Verification items for the finished model (mm, model axes). A direction names the side the tool comes from. Round coordinates to 2 decimals unless told otherwise and drop trailing zeros. Loops run counter-clockwise (first coordinate to the right, second up) from the corner with the lowest first, then second, coordinate; pieces in that order, holes last. Notation, with made-up numbers: (3.5, 25.25) -> (47.5, 25.25) arc R27 cw to (47.5, 57.25) -> close; hole circle Ø10 at (70.5, -29). An arc over 180 degrees is marked (long way). Write item = value, one per line.
```python
from build123d import *

# Parameters (mm, degrees)
BOSS_EXTRUDE1_DEPTH             = 20
SKETCH6_W                       = 25
SKETCH6_H                       = 20
BOSS_EXTRUDE5_DEPTH             = 5.5
BOSS_EXTRUDE11_START            = -20
BOSS_EXTRUDE11_DEPTH            = 34
SKETCH4_R                       = 2
CUT_EXTRUDE1_DEPTH              = 10
BOSS_EXTRUDE13_DEPTH            = 12
FILLET11_START                  = 14.0499999
FILLET11_DEPTH                  = 7.9500001
FILLET11_START_2                = -14.996842371
FILLET11_2_DEPTH                = 30.996842371
SKETCH22_R                      = 2
CUT_EXTRUDE6_DEPTH              = 10
CHAMFER1_SIZE                   = 14
SKETCH26_W                      = 22
SKETCH26_H                      = 20
BOSS_EXTRUDE14_DEPTH            = 11
CUT_EXTRUDE7_DEPTH              = 2.5
CUT_EXTRUDE8_REACH              = 65.92
SKETCH27_R                      = 4
SKETCH27_R_2                    = 1.15
SKETCH27_R_3                    = 1.6
CUT_EXTRUDE9_DEPTH              = 2.5
BOSS_EXTRUDE15_DEPTH            = 1
BOSS_EXTRUDE15_DEPTH_BACK       = 2
SKETCH31_R                      = 4
SKETCH31_R_2                    = 1.65
SKETCH32_R                      = 2.85
SKETCH32_R_2                    = 2.25
CUT_EXTRUDE12_DEPTH             = 7
CUT_EXTRUDE12_DIRECTION_2_REACH = 61.046
SKETCH33_R                      = 3.8
BOSS_EXTRUDE17_DEPTH            = 7
FILLET17_R                      = 1
CUT_EXTRUDE13_DEPTH             = 14
SKETCH36_R                      = 2
CUT_EXTRUDE14_DEPTH             = 10
FILLET18_R                      = 10
CUT_EXTRUDE16_REACH             = 67.49
SKETCH37_W                      = 5.717933373
SKETCH37_H                      = 6
CHAMFER2_SIZE                   = 7
SKETCH38_W                      = 10
SKETCH38_H                      = 20
CUT_EXTRUDE17_DEPTH             = 4
CUT_EXTRUDE19_REACH             = 59.527
SKETCH39_W                      = 10
SKETCH39_H                      = 5


with BuildPart() as part:
    # Sketch1 → Boss-Extrude1 (new body)
    with BuildSketch(Plane(origin=(0, 0, 0), x_dir=(1, 0, 0), z_dir=(0, 1, 0))):
        Polygon((-15.5, -37), (-10, -37), (-10, 4), (11, 4), (11, -37), (18, -37), (18, -27), (21, -19), (21, 10), (-15.5, 10), align=None)
    extrude(amount=BOSS_EXTRUDE1_DEPTH)

    # Sketch6 → Boss-Extrude5 (add)
    with BuildSketch(Plane.ZY.offset(15.5)):
        with Locations((2.5, 10)):
            Rectangle(SKETCH6_W, SKETCH6_H)
    extrude(amount=BOSS_EXTRUDE5_DEPTH)

    # Sketch20 → Boss-Extrude11 (add)
    with BuildSketch(Plane(origin=(0, 20, 0), x_dir=(1, 0, 0), z_dir=(0, 1, 0)).offset(BOSS_EXTRUDE11_START)):
        Polygon((-21, 6.554166441), (14, 6.554166441), (14, -16.445833559), (21.006315459, -12.400735443), (21.006315459, 10.282066627), (15.003157729, 18.901571597), (-14.996842271, 18.901571597), (-21, 10.282066627), align=None)
    extrude(amount=BOSS_EXTRUDE11_DEPTH)

    # Sketch4 → Cut-Extrude1 (cut)
    with BuildSketch(Plane(origin=(0, 20, 0), x_dir=(1, 0, 0), z_dir=(0, 1, 0))):
        with Locations(Location((-4.375, 8, 0), (0, 0, 270))):
            Circle(SKETCH4_R)
        with Locations(Location((5.375, 8, 0), (0, 0, 270))):
            Circle(SKETCH4_R)
    extrude(amount=-CUT_EXTRUDE1_DEPTH, mode=Mode.SUBTRACT)

    # Sketch24 → Boss-Extrude13 (add)
    with BuildSketch(Plane(origin=(0, 34, 0), x_dir=(1, 0, 0), z_dir=(0, 1, 0))):
        with BuildLine():
            Line((-14.996842271, 18.901571597), (-14.420936492, 19.728473528))
            ThreePointArc((-14.420936492, 19.728473528), (-3.81756267, 26.467738085), (8.613124034, 24.643662635))
            ThreePointArc((8.613124034, 24.643662635), (12.140366622, 22.142331504), (15.003157729, 18.901571597))
            Line((15.003157729, 18.901571597), (21.006315459, 10.282066627))
            Line((21.006315459, 10.282066627), (21.006315459, 6.554166441))
            Line((21.006315459, 6.554166441), (-21, 6.554166441))
            Line((-21, 6.554166441), (-21, 10.282066627))
            Line((-21, 10.282066627), (-14.996842271, 18.901571597))
        make_face()
    extrude(amount=-BOSS_EXTRUDE13_DEPTH)

    # Fillet11: read off the stored shape, not the designer's step
    # Fillet11 outline → Fillet11 (add)
    with BuildSketch(Plane(origin=(0, 0, 0), x_dir=(1, 0, 0), z_dir=(0, 1, 0)).offset(FILLET11_START)):
        with BuildLine():
            Line((-14.996842271, 18.901571597), (15.003161757, 18.901565813))
            ThreePointArc((15.003161757, 18.901565813), (12.140369243, 22.142329149), (8.613124034, 24.643662635))
            ThreePointArc((8.613124034, 24.643662635), (-3.81756267, 26.467738085), (-14.420936492, 19.728473528))
            Line((-14.420936492, 19.728473528), (-14.996842271, 18.901571597))
        make_face()
    extrude(amount=FILLET11_DEPTH)

    # Fillet11 2 outline → Fillet11 2 (cut)
    with BuildSketch(Plane.YZ.offset(FILLET11_START_2)):
        with BuildLine():
            Line((22, -28), (22, -26.851571597))
            ThreePointArc((22, -26.851571597), (19.67149891, -21.230072687), (14.05, -18.901571597))
            Line((14.05, -18.901571597), (14.0499999, -28))
            Line((14.0499999, -28), (22, -28))
        make_face()
    extrude(amount=FILLET11_2_DEPTH, mode=Mode.SUBTRACT)

    # Sketch22 → Cut-Extrude6 (cut)
    with BuildSketch(Plane(origin=(0, 34, 0), x_dir=(1, 0, 0), z_dir=(0, 1, 0))):
        with Locations(Location((-14.720302421, 13.351367671, 0), (0, 0, 270))):
            Circle(SKETCH22_R)
        with Locations(Location((-3.067324575, 22.581252689, 0), (0, 0, 270))):
            Circle(SKETCH22_R)
    extrude(amount=-CUT_EXTRUDE6_DEPTH, mode=Mode.SUBTRACT)

    # Chamfer1
    chamfer1_edges = [part.edges().sort_by_distance(p)[0] for p in [
        (17.503157729, 34, 14.423284501),
    ]]
    chamfer(chamfer1_edges, length=CHAMFER1_SIZE)

    # Sketch26 → Boss-Extrude14 (add)
    with BuildSketch(Plane.ZY.offset(21)):
        with Locations((26, 10)):
            Rectangle(SKETCH26_W, SKETCH26_H)
    extrude(amount=-BOSS_EXTRUDE14_DEPTH)

    # Sketch25 → Cut-Extrude7 (cut)
    with BuildSketch(Plane.ZY.offset(21)):
        with BuildLine():
            Line((11.868890963, 14.931194411), (31.150048263, 18.330982662))
            ThreePointArc((31.150048263, 18.330982662), (35.639064994, 15.187739308), (32.49582164, 10.698722576))
            Line((32.49582164, 10.698722576), (13.21466434, 7.298934325))
            ThreePointArc((13.21466434, 7.298934325), (-1.168124774, 8.697638667), (11.868890963, 14.931194411))
        make_face()
    extrude(amount=-CUT_EXTRUDE7_DEPTH, mode=Mode.SUBTRACT)

    # Sketch27 → Cut-Extrude8 (cut, up to next)
    with BuildSketch(Plane.ZY.offset(18.5), mode=Mode.PRIVATE) as cut_extrude8_sk1:
        with Locations((6.217933373, 10)):
            Circle(SKETCH27_R)
    cut_extrude8_tool1 = extrude(cut_extrude8_sk1.sketch, amount=-CUT_EXTRUDE8_REACH, mode=Mode.PRIVATE) & part.part
    # Sketch27 → Cut-Extrude8 (cut, up to next)
    with BuildSketch(Plane.ZY.offset(18.5), mode=Mode.PRIVATE) as cut_extrude8_sk2:
        with Locations((15.08120315, 11.562833599)):
            Circle(SKETCH27_R_2)
    cut_extrude8_tool2 = extrude(cut_extrude8_sk2.sketch, amount=-CUT_EXTRUDE8_REACH, mode=Mode.PRIVATE) & part.part
    # Sketch27 → Cut-Extrude8 (cut, up to next)
    with BuildSketch(Plane.ZY.offset(18.5), mode=Mode.PRIVATE) as cut_extrude8_sk3:
        with Locations((29.853319446, 14.167556264)):
            Circle(SKETCH27_R_3)
    cut_extrude8_tool3 = extrude(cut_extrude8_sk3.sketch, amount=-CUT_EXTRUDE8_REACH, mode=Mode.PRIVATE) & part.part
    add(cut_extrude8_tool1.solids().sort_by_distance((-18.5, 10, 6.217933))[0], mode=Mode.SUBTRACT)
    add(cut_extrude8_tool2.solids().sort_by_distance((-18.5, 11.562834, 15.081203))[0], mode=Mode.SUBTRACT)
    add(cut_extrude8_tool3.solids().sort_by_distance((-18.5, 14.167556, 29.853319))[0], mode=Mode.SUBTRACT)

    # Sketch28 → Cut-Extrude9 (cut)
    with BuildSketch(Plane.ZY.offset(21)):
        Polygon((-0.028318142, 0.777915528), (-3.197748963, 15.950413947), (10.506443157, 18.813125656), (17.248705835, 15.879800924), (18.680061689, 9.027704864), (13.675873978, 3.640627238), align=None)
    extrude(amount=-CUT_EXTRUDE9_DEPTH, mode=Mode.SUBTRACT)

    # Sketch31 → Boss-Extrude15 (add, two sides: drawn at the far end of the back side and taken through both)
    with BuildSketch(Plane.ZY.offset(18.5).offset(-BOSS_EXTRUDE15_DEPTH_BACK)):
        with Locations((6.217933373, 10)):
            Circle(SKETCH31_R)
        with Locations((6.217933373, 10)):
            Circle(SKETCH31_R_2, mode=Mode.SUBTRACT)
    extrude(amount=BOSS_EXTRUDE15_DEPTH + BOSS_EXTRUDE15_DEPTH_BACK)

    # Sketch32 → Cut-Extrude12 (cut)
    with BuildSketch(Plane(origin=(-10, 0, 0), x_dir=(0, 0, -1), z_dir=(1, 0, 0))):
        with Locations((-29.853319446, 14.167556264)):
            Circle(SKETCH32_R)
        with Locations((-15.08120315, 11.562833599)):
            Circle(SKETCH32_R_2)
    extrude(amount=-CUT_EXTRUDE12_DEPTH, mode=Mode.SUBTRACT)

    # Sketch32 → Cut-Extrude12 direction 2 (cut, up to next)
    with BuildSketch(Plane(origin=(-10, 0, 0), x_dir=(0, 0, -1), z_dir=(1, 0, 0)), mode=Mode.PRIVATE) as cut_extrude12_direction_2_sk1:
        with Locations((-29.853319446, 14.167556264)):
            Circle(SKETCH32_R)
    cut_extrude12_direction_2_tool1 = extrude(cut_extrude12_direction_2_sk1.sketch, amount=CUT_EXTRUDE12_DIRECTION_2_REACH, mode=Mode.PRIVATE) & part.part
    # Sketch32 → Cut-Extrude12 direction 2 (cut, up to next)
    with BuildSketch(Plane(origin=(-10, 0, 0), x_dir=(0, 0, -1), z_dir=(1, 0, 0)), mode=Mode.PRIVATE) as cut_extrude12_direction_2_sk2:
        with Locations((-15.08120315, 11.562833599)):
            Circle(SKETCH32_R_2)
    cut_extrude12_direction_2_tool2 = extrude(cut_extrude12_direction_2_sk2.sketch, amount=CUT_EXTRUDE12_DIRECTION_2_REACH, mode=Mode.PRIVATE) & part.part
    add(cut_extrude12_direction_2_tool1.solids().sort_by_distance((-10, 14.167556, 29.853319))[0], mode=Mode.SUBTRACT)
    add(cut_extrude12_direction_2_tool2.solids().sort_by_distance((-10, 11.562834, 15.081203))[0], mode=Mode.SUBTRACT)

    # Sketch33 → Boss-Extrude17 (add)
    with BuildSketch(Plane(origin=(21.006315459, 0, 0), x_dir=(0, 0, -1), z_dir=(1, 0, 0))):
        with Locations((-6.217933373, 10)):
            Circle(SKETCH33_R)
    extrude(amount=BOSS_EXTRUDE17_DEPTH)

    # Fillet17
    fillet17_edges = [part.edges().sort_by_distance(p)[0] for p in [
        (28.006315459, 10, 10.017933373),
    ]]
    fillet(fillet17_edges, radius=FILLET17_R)

    # Sketch35 → Cut-Extrude13 (cut)
    with BuildSketch(Plane(origin=(0, 34, 0), x_dir=(1, 0, 0), z_dir=(0, 1, 0))):
        with BuildLine():
            Line((-19.79995418, 6.554166441), (14, 6.554166441))
            Line((14, 6.554166441), (14, 12.554166441))
            Line((14, 12.554166441), (-9.802737675, 12.554166441))
            ThreePointArc((-9.802737675, 12.554166441), (-11.071315957, 11.28171537), (-12.284990593, 9.956794065))
            ThreePointArc((-12.284990593, 9.956794065), (-15.675255632, 7.444453939), (-19.79995418, 6.554166441))
        make_face()
    extrude(amount=-CUT_EXTRUDE13_DEPTH, mode=Mode.SUBTRACT)

    # Sketch36 → Cut-Extrude14 (cut)
    with BuildSketch(Plane.XY.offset(37)):
        with Locations((-15.25, 14)):
            Circle(SKETCH36_R)
        with Locations((14.5, 10)):
            Circle(SKETCH36_R)
        with Locations((-15.25, 4)):
            Circle(SKETCH36_R)
    extrude(amount=-CUT_EXTRUDE14_DEPTH, mode=Mode.SUBTRACT)

    # Fillet18
    fillet18_edges = [part.edges().sort_by_distance(p)[0] for p in [
        (0.003157729, 0, -18.901571597),
    ]]
    fillet(fillet18_edges, radius=FILLET18_R)

    # Sketch37 → Cut-Extrude16 (cut, up to next)
    with BuildSketch(Plane(origin=(21, 0, 0), x_dir=(0, 0, -1), z_dir=(1, 0, 0)), mode=Mode.PRIVATE) as cut_extrude16_sk1:
        with Locations((1.141033313, 10)):
            Rectangle(SKETCH37_W, SKETCH37_H)
    cut_extrude16_tool1 = extrude(cut_extrude16_sk1.sketch, amount=-CUT_EXTRUDE16_REACH, mode=Mode.PRIVATE) & part.part
    add(cut_extrude16_tool1.solids().sort_by_distance((21, 10, -1.141033))[0], mode=Mode.SUBTRACT)

    # Chamfer2
    chamfer2_edges = [part.edges().sort_by_distance(p)[0] for p in [
        (11, 10, 1.717933373),
    ]]
    chamfer(chamfer2_edges, length=CHAMFER2_SIZE)

    # Sketch38 → Cut-Extrude17 (cut)
    with BuildSketch(Plane.XZ):
        with Locations((0.5, -14)):
            Rectangle(SKETCH38_W, SKETCH38_H)
    extrude(amount=-CUT_EXTRUDE17_DEPTH, mode=Mode.SUBTRACT)

    # Sketch39 → Cut-Extrude19 (cut, up to next)
    with BuildSketch(Plane(origin=(0, 34, 0), x_dir=(1, 0, 0), z_dir=(0, 1, 0)), mode=Mode.PRIVATE) as cut_extrude19_sk1:
        with Locations((0.5, 15.054166441)):
            Rectangle(SKETCH39_W, SKETCH39_H)
    cut_extrude19_tool1 = extrude(cut_extrude19_sk1.sketch, amount=-CUT_EXTRUDE19_REACH, mode=Mode.PRIVATE) & part.part
    add(cut_extrude19_tool1.solids().sort_by_distance((0.5, 34, -15.054166))[0], mode=Mode.SUBTRACT)


solid = part.part
```
(1) Draft check along Z on faces 1 (the face through (0, 34, -20)), 2 (the face through (-3.642, 27.5, -26.504)), 3 (the face through (-17.979, 8.996, 4.909)), 4 (the face through (10, 27, -12.554)). Enter one of: released by +Z, released by -Z, zero draft, split by the parting line, or undercut.
Filled sheet:
face_1 = zero draft
face_2 = released by -Z
face_3 = undercut
face_4 = released by +Z
(2) Sectioned sample at C-C, the plane z = -8. Record the cut outline in (x, y) (3 decimals), and give its area (3 significant figures).
Filled sheet:
outline = (-21, 0) -> (-4.5, 0) -> (-4.5, 4) -> (5.5, 4) -> (5.5, 0) -> (21.006, 0) -> (21.006, 34) -> (14, 34) -> (14, 20) -> (7.375, 20) -> (7.375, 10) -> (3.375, 10) -> (3.375, 20) -> (-2.375, 20) -> (-2.375, 10) -> (-6.375, 10) -> (-6.375, 20) -> (-14.621, 20) -> (-14.621, 34) -> (-21, 34) -> close
area = 908 mm2
(3) Sectioned sample at A-A, the plane z = 24. Record the cut outline in (x, y) (3 decimals), and give its area (3 significant figures).
Filled sheet:
outline = (-21, 0) -> (-10, 0) -> (-10, 20) -> (-21, 20) -> (-21, 17.07) -> (-18.5, 17.07) -> (-18.5, 9.201) -> (-21, 9.201) -> close; (11, 0) -> (19.125, 0) -> (19.125, 20) -> (11, 20) -> close
area = 363 mm2
(4) Set-up check for faces 5 (the face through (-14, 20, 12)), 6 (the face through (-17.203, 13.567, 27.548)), 7 (the face through (-2.98, 29.07, -24.58)), 8 (the face through (-19.768, 17.088, 24.102)): record each of +Z, -Z, +X, -X, +Y, -Y from which the full face is reachable in a straight line by a thin tool's end or side.
Filled sheet:
face_5 = +Z, +Y
face_6 = +Z
face_7 = +Y
face_8 = -X
(5) Go/stop test with flat-tipped pins: pin 1 Ø2.5 at (y, z) = (10, 7.5) entering from -X; pin 2 Ø6 at (x, y) = (-8, 29.5) entering from +Z; pin 3 Ø2 at (x, y) = (-14.5, 14) entering from +Z; pin 4 Ø12 at (y, z) = (30, 21.5) entering from +X. Record where each tip stops, or that it passes through.
Filled sheet:
pin_1 = -19.5
pin_2 = -11.36
pin_3 = 27
pin_4 = through
(6) Sectioned sample at B-B, the plane y = 25. Record the cut outline in (x, z) (3 decimals), and give its area (3 significant figures).
Filled sheet:
outline = (-21, -10.282) -> (-14.421, -19.728) arc R18.027 ccw to (8.613, -24.644) arc R18.809 ccw to (15.003, -18.902) -> (21.006, -10.282) -> (21.006, 6.627) -> (14, 10.672) -> (14, -12.554) -> (5.5, -12.554) -> (5.5, -17.554) -> (-4.5, -17.554) -> (-4.5, -12.554) -> (-9.803, -12.554) arc R42.51 cw to (-12.285, -9.957) arc R10 ccw to (-19.8, -6.554) -> (-21, -6.554) -> close; hole circle Ø4 at (-14.72, -13.351); hole circle Ø4 at (-3.067, -22.581)
area = 504 mm2
(7) Material ranges on probe 1 along Y at (x, z) = (-15.25, 35.5); probe 2 along Y at (x, z) = (14.5, 34); probe 3 along X at (y, z) = (14, -2.5), recorded low to high. Write a range as from..to.
Filled sheet:
probe_1 = 0..2, 6..12, 16..20
probe_2 = 0..8, 12..20
probe_3 = -18.5..-10, 11..21.01
